```python
from build123d import *

# Parameters (mm, degrees)
CUT_EXTRUDE1_DEPTH = 0.75
FILLET1_R          = 0.125


with BuildPart() as part:
    # Sketch1 → Revolve1 (revolve)
    with BuildSketch(Plane(origin=(0, 0, 0), x_dir=(0, 0, -1), z_dir=(1, 0, 0))):
        with BuildLine():
            Line((0, 1.5), (-1.5, 1.5))
            ThreePointArc((-1.5, 1.5), (-1.978515811, 0.925250119), (-2.3, 0.25))
            Line((-2.3, 0.25), (-2.155662433, 0))
            Line((-2.155662433, 0), (-1, 0))
            Line((-1, 0), (-1, -20))
            Line((-1, -20), (0, -20))
            Line((0, -20), (0, 1.5))
        make_face()
    revolve(axis=Axis((0, -20, 0), (0, 1, 0)))

    # Sketch2 → Cut-Extrude1 (cut)
    with BuildSketch(Plane(origin=(0, 1.5, 0), x_dir=(1, 0, 0), z_dir=(0, 1, 0))):
        Polygon((0, 1.154700538), (-1, 0.577350269), (-1, -0.577350269), (0, -1.154700538), (1, -0.577350269), (1, 0.577350269), align=None)
    extrude(amount=-CUT_EXTRUDE1_DEPTH, mode=Mode.SUBTRACT)

    # Fillet1
    fillet1_edges = [part.edges().sort_by_distance(p)[0] for p in [
        (0.5, 1.5, -0.866025404),
        (-0.5, 1.5, -0.866025404),
        (-1, 1.5, 0),
        (-0.5, 1.5, 0.866025404),
        (0.5, 1.5, 0.866025404),
        (1, 1.5, 0),
        (0, 1.5, -1.5),
    ]]
    fillet(fillet1_edges, radius=FILLET1_R)


solid = part.part
```
Source: CAD feature listing. Evaluate the final solid. Frame: model axes, mm. Coordinates: 2 decimals unless noted, no trailing zeros. Loops run counter-clockwise (first coordinate to the right, second up) from the corner with the lowest first, then second, coordinate; pieces in that order, holes last. Notation, with made-up numbers: (86.5, 69.25) - (118.5, 69.25) arc R17 cw to (118.5, 81.25) - close; hole circle Ø7 at (18.25, 74.5). An arc over 180 degrees is marked (long way). Answer as CSV lines item,"result".
1. Section A-A (y = -9.5). Return loops of the section in (x, z).
Established:
outline,"circle Ø2 at (0, 0)"
2. Ray query, line 1 (Y direction, x = -0.7, z = 0.45); line 2 (Z direction, x = -0.1, y = -3.75); line 3 (Y direction, x = -1.2, z = -0.75). Return the intervals inside material, ascending.
Established:
line 1,"y = -20 to 0.75"
line 2,"z = -0.99 to 0.99"
line 3,"y = 0 to 1.5"
3. Contact query for flat-ended pins moving along their axis: pin 1 (0.5 mm diameter, centred on y = 1, z = 0, fed in from -X); pin 2 (0.6 mm diameter, centred on x = 0, z = 0, fed in from +Y); pin 3 (1 mm diameter, centred on y = -9, z = 1, fed in from -X); pin 4 (1.5 mm diameter, centred on x = 0.5, z = -2, fed in from +Y). Output: stop coordinate, or through.
Established:
pin 1,"stops at x = -2.08"
pin 2,"stops at y = 0.75"
pin 3,"stops at x = -0.87"
pin 4,"stops at y = 1.5"
4. Mould query, pull axis X, two halves, no side actions, for faces 1 (the cylindrical face through (-1, -10, 0)), 2 (the flat face through (1, 0, 1)), 3 (the flat face through (0, 0.75, 0)). Classes: released by +X, released by -X, zero draft, split by the parting line, or undercut.
Established:
face 1,"split by the parting line"
face 2,"zero draft"
face 3,"undercut"
